```python
from build123d import *

# Parameters (mm, degrees)
F0_W         = 50.8
F0_H         = 30
F1_DEPTH     = 10
F2_W         = 3
F2_H         = 26
F2_W_2       = 11.5
F2_H_2       = 1.5
F3_DEPTH     = 8
F4_T1_DEPTH  = 13
F4_T3_DEPTH  = 26
F4_T5_DEPTH  = 46.8
F4_S9_W      = 2
F4_S9_H      = 2
F4_T10_DEPTH = 2
F4_S15_W     = 2
F4_S15_H     = 2
F4_T16_DEPTH = 2
F4_S21_W     = 2
F4_S21_H     = 2
F4_T22_DEPTH = 2
F4_S27_W     = 2
F4_S27_H     = 2
F4_T28_DEPTH = 2


# Not quite as in the source:
# - a fillet or chamfer that OpenCascade refuses, or shapes differently, is made with other operations: its cross-section is extruded or revolved along the edge and cut away or added


with BuildPart() as f1:
    # F0 (on Top) → F1 (new body)
    with BuildSketch(Plane.XY):
        Rectangle(F0_W, F0_H)
    extrude(amount=F1_DEPTH)

    # F2 (on Top) → F3 (cut)
    with BuildSketch(Plane.XY):
        with Locations((-7.3340023962, 0.1232437862)):
            Rectangle(F2_W, F2_H)
        with Locations((-11.9503338486, 0.091059359)):
            Rectangle(F2_W, F2_H)
        with Locations((-16.8786235154, 0.0321844273)):
            Rectangle(F2_W, F2_H)
        with Locations((-21.4949549678, 0)):
            Rectangle(F2_W, F2_H)
        with Locations((5.75, 4.3395428155)):
            Rectangle(F2_W_2, F2_H_2)
        with Locations((5.75, 6.9914316775)):
            Rectangle(F2_W_2, F2_H_2)
        with Locations((5.75, 9.7213549241)):
            Rectangle(F2_W_2, F2_H_2)
        with Locations((5.75, 12.3732437862)):
            Rectangle(F2_W_2, F2_H_2)
        with Locations((5.75, 1.6359822841)):
            Rectangle(F2_W_2, F2_H_2)
        with Locations((5.75, -1.0159065779)):
            Rectangle(F2_W_2, F2_H_2)
        with Locations((5.75, -3.7458298245)):
            Rectangle(F2_W_2, F2_H_2)
        with Locations((5.75, -6.3977186866)):
            Rectangle(F2_W_2, F2_H_2)
    extrude(amount=F3_DEPTH, mode=Mode.SUBTRACT)

    # F4: fillet of radius 2 on 8 edges, made by hand

    # F4_s2 → F4_t1 (cut)
    with BuildSketch(Plane.XY.offset(2)):
        with BuildLine():
            ThreePointArc((25.4, 13), (24.8142135624, 14.4142135624), (23.4, 15))
            Line((23.4, 15), (25.4, 15))
            Line((25.4, 15), (25.4, 13))
        make_face()
        with BuildLine():
            ThreePointArc((25.4, -13), (24.8142135624, -14.4142135624), (23.4, -15))
            Line((23.4, -15), (25.4, -15))
            Line((25.4, -15), (25.4, -13))
        make_face()
        with BuildLine():
            ThreePointArc((-23.4, -15), (-24.8142135624, -14.4142135624), (-25.4, -13))
            Line((-25.4, -13), (-25.4, -15))
            Line((-25.4, -15), (-23.4, -15))
        make_face()
        with BuildLine():
            ThreePointArc((-23.4, 15), (-24.8142135624, 14.4142135624), (-25.4, 13))
            Line((-25.4, 13), (-25.4, 15))
            Line((-25.4, 15), (-23.4, 15))
        make_face()
    extrude(amount=F4_T1_DEPTH, mode=Mode.SUBTRACT)

    # F4_s4 → F4_t3 (cut)
    with BuildSketch(Plane.XZ.offset(-13)):
        with BuildLine():
            ThreePointArc((25.4, 2), (24.8142135624, 0.5857864376), (23.4, 0))
            Line((23.4, 0), (25.4, 0))
            Line((25.4, 0), (25.4, 2))
        make_face()
        with BuildLine():
            ThreePointArc((-23.4, 0), (-24.8142135624, 0.5857864376), (-25.4, 2))
            Line((-25.4, 2), (-25.4, 0))
            Line((-25.4, 0), (-23.4, 0))
        make_face()
    extrude(amount=F4_T3_DEPTH, mode=Mode.SUBTRACT)

    # F4_s6 → F4_t5 (cut)
    with BuildSketch(Plane.YZ.offset(-23.4)):
        with BuildLine():
            ThreePointArc((-15, 2), (-14.4142135624, 0.5857864376), (-13, 0))
            Line((-13, 0), (-15, 0))
            Line((-15, 0), (-15, 2))
        make_face()
        with BuildLine():
            ThreePointArc((15, 2), (14.4142135624, 0.5857864376), (13, 0))
            Line((13, 0), (15, 0))
            Line((15, 0), (15, 2))
        make_face()
    extrude(amount=F4_T5_DEPTH, mode=Mode.SUBTRACT)


with BuildPart() as f4_tool8:
    # F4_s9 → F4_t10 (new body)
    with BuildSketch(Plane.YZ.offset(23.4)):
        with Locations((14, 1)):
            Rectangle(F4_S9_W, F4_S9_H)
    extrude(amount=F4_T10_DEPTH)

    # F4_s11 → F4_t12 (revolve, cut)
    with BuildSketch(Plane(origin=(23.4, 13, 2), x_dir=(0, -0.7071067812, 0.7071067812), z_dir=(0, 0.7071067812, 0.7071067812))):
        with BuildLine():
            ThreePointArc((0, -2), (2, 0), (0, 2))
            Line((0, 2), (0, -2))
        make_face()
    revolve(axis=Axis((23.4, 13, 2), (1, 0, 0)), mode=Mode.SUBTRACT)


with BuildPart() as f1_1:
    add(f1.part)

    # F4_t7: cut F4_tool8
    add(f4_tool8.part, mode=Mode.SUBTRACT)


with BuildPart() as f4_tool14:
    # F4_s15 → F4_t16 (new body)
    with BuildSketch(Plane.YZ.offset(23.4)):
        with Locations((-14, 1)):
            Rectangle(F4_S15_W, F4_S15_H)
    extrude(amount=F4_T16_DEPTH)

    # F4_s17 → F4_t18 (revolve, cut)
    with BuildSketch(Plane(origin=(23.4, -13, 2), x_dir=(0, 0.7071067812, 0.7071067812), z_dir=(0, 0.7071067812, -0.7071067812))):
        with BuildLine():
            ThreePointArc((0, -2), (2, 0), (0, 2))
            Line((0, 2), (0, -2))
        make_face()
    revolve(axis=Axis((23.4, -13, 2), (1, 0, 0)), mode=Mode.SUBTRACT)


with BuildPart() as f1_2:
    add(f1_1.part)

    # F4_t13: cut F4_tool14
    add(f4_tool14.part, mode=Mode.SUBTRACT)


with BuildPart() as f4_tool20:
    # F4_s21 → F4_t22 (new body)
    with BuildSketch(Plane.XZ.offset(13)):
        with Locations((-24.4, 1)):
            Rectangle(F4_S21_W, F4_S21_H)
    extrude(amount=F4_T22_DEPTH)

    # F4_s23 → F4_t24 (revolve, cut)
    with BuildSketch(Plane(origin=(-23.4, -13, 2), x_dir=(0.7071067812, 0, 0.7071067812), z_dir=(0.7071067812, 0, -0.7071067812))):
        with BuildLine():
            ThreePointArc((0, -2), (2, 0), (0, 2))
            Line((0, 2), (0, -2))
        make_face()
    revolve(axis=Axis((-23.4, -13, 2), (0, -1, 0)), mode=Mode.SUBTRACT)


with BuildPart() as f1_3:
    add(f1_2.part)

    # F4_t19: cut F4_tool20
    add(f4_tool20.part, mode=Mode.SUBTRACT)


with BuildPart() as f4_tool26:
    # F4_s27 → F4_t28 (new body)
    with BuildSketch(Plane.XZ.offset(-13)):
        with Locations((-24.4, 1)):
            Rectangle(F4_S27_W, F4_S27_H)
    extrude(amount=-F4_T28_DEPTH)

    # F4_s29 → F4_t30 (revolve, cut)
    with BuildSketch(Plane(origin=(-23.4, 13, 2), x_dir=(0.7071067812, 0, 0.7071067812), z_dir=(-0.7071067812, 0, 0.7071067812))):
        with BuildLine():
            ThreePointArc((0, -2), (2, 0), (0, 2))
            Line((0, 2), (0, -2))
        make_face()
    revolve(axis=Axis((-23.4, 13, 2), (0, 1, 0)), mode=Mode.SUBTRACT)


with BuildPart() as f1_4:
    add(f1_3.part)

    # F4_t25: cut F4_tool26
    add(f4_tool26.part, mode=Mode.SUBTRACT)


solid = f1_4.part
```
Input: part model. Units: mm. Frame: model coordinates. Give positions to 0.01 mm unless a question says otherwise; leave off trailing zeros. Order: outer loops, then holes, each group sorted by start corner. A loop starts at its lowest first (then second) coordinate and runs counter-clockwise, first axis right, second up. Notation, with made-up numbers: M -15,9.5 L 38,9.5 A23 cw 38,25.5 Z; hole C 40.5,35 d6. An arc over 180 degrees is marked long. Return JSON: item names as keys, results as strings.
Item 1: Cut plane B-B (z = 3.5). State how many separate pieces and enclosed holes the cut face has, then the cut area to 3 significant figures.
Solutions:
{"separate pieces": "1", "enclosed holes": "12", "area": "1,070 mm^2"}
Item 2: First-contact query: P1, Ø1.6, axis at x = 6, y = -6.5, coming from the -Z side; P2, Ø1.5, axis at x = -21, y = -1, coming from the -Z side. Flat tips, straight axial feed; report the tip coordinate or a pass-through.
Solutions:
{"P1": "z = 0", "P2": "z = 8"}
Item 3: Cut plane A-A (y = 9.5). Return loops of the section in (x, z), then the cut area to 3 significant figures.
Solutions:
{"outline": "M -25.4,2 A2 ccw -23.4,0 L -22.99,0 L -22.99,8 L -19.99,8 L -19.99,0 L -18.38,0 L -18.38,8 L -15.38,8 L -15.38,0 L -13.45,0 L -13.45,8 L -10.45,8 L -10.45,0 L -8.83,0 L -8.83,8 L -5.83,8 L -5.83,0 L 0,0 L 0,8 L 11.5,8 L 11.5,0 L 23.4,0 A2 ccw 25.4,2 L 25.4,10 L -25.4,10 Z", "area": "318 mm^2"}
Item 4: Ray query, probe 1 along X at (y, z) = (6, 6.75); probe 2 along X at (y, z) = (-1, 2); probe 3 along X at (y, z) = (1, 1.5). Return the intervals inside material, ascending.
Solutions:
{"probe 1": "-25.4 to -22.99, -19.99 to -18.38, -15.38 to -13.45, -10.45 to -8.83, -5.83 to 25.4", "probe 2": "-25.4 to -22.99, -19.99 to -18.38, -15.38 to -13.45, -10.45 to -8.83, -5.83 to 0, 11.5 to 25.4", "probe 3": "-25.34 to -22.99, -19.99 to -18.38, -15.38 to -13.45, -10.45 to -8.83, -5.83 to 0, 11.5 to 25.34"}
Item 5: Pull-direction query (Y, two-part tool) for faces 1 (the flat face through (11.5, 4, 4)), 2 (the flat face through (0, -15, 6)); classes: +Y half, -Y half, draft (parallel to the pull), parting line (faces both ways), or undercut.
Solutions:
{"face 1": "undercut", "face 2": "-Y half"}
Item 6: Cut plane C-C (y = -2.5). Return loops of the section in (x, z).
Solutions:
{"outline": "M -25.4,2 A2 ccw -23.4,0 L -22.99,0 L -22.99,8 L -19.99,8 L -19.99,0 L -18.38,0 L -18.38,8 L -15.38,8 L -15.38,0 L -13.45,0 L -13.45,8 L -10.45,8 L -10.45,0 L -8.83,0 L -8.83,8 L -5.83,8 L -5.83,0 L 23.4,0 A2 ccw 25.4,2 L 25.4,10 L -25.4,10 Z"}
